from build123d import *

# Parameters (mm, degrees)
SKETCH3_W           = 302.8427
SKETCH3_H           = 302.8427
BOSS_EXTRUDE1_DEPTH = 790
BOSS_EXTRUDE1_DRAFT = -3
SKETCH6_W           = 200
SKETCH6_H           = 200
CUT_EXTRUDE3_DEPTH  = 790
CUT_EXTRUDE3_DRAFT  = 3
SKETCH7_W           = 250
SKETCH7_H           = 250
SKETCH7_R           = 2.5
SKETCH7_W_2         = 200
SKETCH7_H_2         = 200
BOSS_EXTRUDE2_DEPTH = 5
SKETCH8_W           = 332.804291268
SKETCH8_H           = 332.804291268
SKETCH8_R           = 2.5
SKETCH8_W_2         = 282.804291268
SKETCH8_H_2         = 282.804291268
BOSS_EXTRUDE3_DEPTH = 5


with BuildPart() as part:
    # Sketch3 → Boss-Extrude1 (with draft: the straight prism first)
    with BuildSketch(Plane.XY.offset(790)):
        Rectangle(SKETCH3_W, SKETCH3_H)
    extrude(amount=-BOSS_EXTRUDE1_DEPTH)
    # Boss-Extrude1: the draft: its side faces are tilted about the plane it starts from
    boss_extrude1_sides = [part.faces().sort_by_distance(p)[0] for p in [
        (0, 151.42135, 395),
        (-151.42135, 0, 395),
        (0, -151.42135, 395),
        (151.42135, 0, 395),
    ]]
    draft(boss_extrude1_sides, Plane.XY.offset(790), BOSS_EXTRUDE1_DRAFT)


with BuildPart() as cut_extrude3_tool:
    # Sketch6 → Cut-Extrude3 (with draft: the straight prism first)
    with BuildSketch(Plane(origin=(0, 0, 0), x_dir=(-1, 0, 0), z_dir=(0, 0, -1))):
        Rectangle(SKETCH6_W, SKETCH6_H)
    extrude(amount=-CUT_EXTRUDE3_DEPTH)
    # Cut-Extrude3: the draft: its side faces are tilted about the plane it starts from
    cut_extrude3_sides = [cut_extrude3_tool.faces().sort_by_distance(p)[0] for p in [
        (0, -100, 395),
        (-100, 0, 395),
        (0, 100, 395),
        (100, 0, 395),
    ]]
    draft(cut_extrude3_sides, Plane(origin=(0, 0, 0), x_dir=(-1, 0, 0), z_dir=(0, 0, -1)), CUT_EXTRUDE3_DRAFT)


with BuildPart() as part_1:
    add(part.part)

    # Cut-Extrude3: cut by cut_extrude3_tool
    add(cut_extrude3_tool.part, mode=Mode.SUBTRACT)

    # Sketch7 → Boss-Extrude2 (add)
    with BuildSketch(Plane(origin=(0, 0, 0), x_dir=(-1, 0, 0), z_dir=(0, 0, -1))):
        Rectangle(SKETCH7_W, SKETCH7_H)
        with Locations((0, -117.5)):
            Circle(SKETCH7_R, mode=Mode.SUBTRACT)
        with Locations((-117.509602183, 117.509602183)):
            Circle(SKETCH7_R, mode=Mode.SUBTRACT)
        with Locations(Location((117.509602183, -117.509602183, 0), (0, 0, 180))):
            Circle(SKETCH7_R, mode=Mode.SUBTRACT)
        with Locations(Location((-117.5, 0, 0), (0, 0, 180))):
            Circle(SKETCH7_R, mode=Mode.SUBTRACT)
        with Locations((-117.509602183, -117.509602183)):
            Circle(SKETCH7_R, mode=Mode.SUBTRACT)
        with Locations(Location((117.509602183, 117.509602183, 0), (0, 0, 180))):
            Circle(SKETCH7_R, mode=Mode.SUBTRACT)
        with Locations((117.5, 0)):
            Circle(SKETCH7_R, mode=Mode.SUBTRACT)
        with Locations((-1.21803637, 117.509602183)):
            Circle(SKETCH7_R, mode=Mode.SUBTRACT)
        Rectangle(SKETCH7_W_2, SKETCH7_H_2, mode=Mode.SUBTRACT)
    extrude(amount=-BOSS_EXTRUDE2_DEPTH)

    # Sketch8 → Boss-Extrude3 (add)
    with BuildSketch(Plane.XY.offset(790)):
        Rectangle(SKETCH8_W, SKETCH8_H)
        with Locations((-158.911747817, 0)):
            Circle(SKETCH8_R, mode=Mode.SUBTRACT)
        with Locations((-158.911747817, 158.911747817)):
            Circle(SKETCH8_R, mode=Mode.SUBTRACT)
        with Locations(Location((158.911747817, -158.911747817, 0), (0, 0, 180))):
            Circle(SKETCH8_R, mode=Mode.SUBTRACT)
        with Locations(Location((0, -158.911747817, 0), (0, 0, 180))):
            Circle(SKETCH8_R, mode=Mode.SUBTRACT)
        with Locations((158.911747817, 158.911747817)):
            Circle(SKETCH8_R, mode=Mode.SUBTRACT)
        with Locations((0, 158.911747817)):
            Circle(SKETCH8_R, mode=Mode.SUBTRACT)
        with Locations(Location((-158.911747817, -158.911747817, 0), (0, 0, 180))):
            Circle(SKETCH8_R, mode=Mode.SUBTRACT)
        with Locations((158.911747817, 0)):
            Circle(SKETCH8_R, mode=Mode.SUBTRACT)
        Rectangle(SKETCH8_W_2, SKETCH8_H_2, mode=Mode.SUBTRACT)
    extrude(amount=-BOSS_EXTRUDE3_DEPTH)


solid = part_1.part
The listing builds one solid part. Answer for the finished solid, in the listing's coordinates (mm). A direction names the side the tool comes from. Give positions to 0.01 mm unless a question says otherwise; leave off trailing zeros. Write each loop counter-clockwise with the first axis right and the second up, starting at its lowest first coordinate (ties: lowest second). Pieces come first, ordered by that corner, then holes. Notation, with made-up numbers: (1.5, 75.5) -> (18.5, 75.5) arc R29 cw to (18.5, 99.5) -> close; hole circle Ø8 at (14.25, 41.25). An arc over 180 degrees is marked (long way). One line per question, with ' | ' between items. Start each with the question number.
1. Section A-A (y = 35) is taken. Determine the outline of the cut face in (x, z), plus the area to 3 significant figures.
2. Section C-C (z = 644) is taken. Determine the outline of the cut face in (x, y).
3. For a pull along Z with two mould halves and no side action, classify faces 1 (the flat face through (-120.544, -1.98, 392.005)), 2 (the flat face through (113, 2, 0)), 3 (the flat face through (-2.116, -131.006, 400.46)) as pulls with the +Z half, pulls with the -Z half, needs draft (parallel to the pull), parting line crosses it, or undercut.
4. Find the intervals of material crossed by probe 1 along Y at (x, z) = (0, 787.8); probe 2 along X at (y, z) = (-32.5, 209); probe 3 along X at (y, z) = (-4.5, 536), in increasing order.
5. For faces 4 (the flat face through (1.98, 120.544, 392.005)), 5 (the flat face through (-2.116, 131.006, 400.46)), 6 (the flat face through (1, 112, 5)), 7 (the flat face through (131.006, -2.116, 400.46)), 8 (the flat face through (-161, 13, 785)), determine the directions among +Z, -Z, +X, -X, +Y, -Y from which every point of the face is accessible in a straight line to the end or side of a thin tool.
6. Given pin 1 Ø4 at (x, z) = (131.5, 556.5) entering from +Y; pin 2 Ø3 at (x, y) = (-158.91, -158.91) entering from +Z; pin 3 Ø6 at (x, y) = (-158.91, 158.91) entering from -Z; pin 4 Ø4 at (x, z) = (42, 2.5) entering from -Y, each flat-ended and moving along its own axis, determine where each tip first touches the part or whether it passes through.
7. Section D-D (z = 207.5) is taken. Determine the outline of the cut face in (x, y), plus the area to 3 significant figures.
Response values:
1) outline: (-166.4, 785) -> (-151.16, 785) -> (-110.28, 5) -> (-125, 5) -> (-125, 0) -> (-100, 0) -> (-100, 5) -> (-100.26, 5) -> (-141.4, 790) -> (-166.4, 790) -> close; (100, 0) -> (125, 0) -> (125, 5) -> (110.28, 5) -> (151.16, 785) -> (166.4, 785) -> (166.4, 790) -> (141.4, 790) -> (100.26, 5) -> (100, 5) -> close | area: 16,100 mm2
2) outline: (-143.77, -143.77) -> (143.77, -143.77) -> (143.77, 143.77) -> (-143.77, 143.77) -> close; hole (-133.75, -133.75) -> (133.75, -133.75) -> (133.75, 133.75) -> (-133.75, 133.75) -> close
3) face 1: pulls with the +Z half | face 2: pulls with the -Z half | face 3: undercut
4) probe 1: -166.4 to -161.41, -156.41 to -141.29, 141.29 to 156.41, 161.41 to 166.4 | probe 2: -120.97 to -110.95, 110.95 to 120.97 | probe 3: -138.11 to -128.09, 128.09 to 138.11
5) face 4: +Z | face 5: +X, -X, +Y | face 6: none | face 7: +X, +Y, -Y | face 8: -Z
6) pin 1: y = 139.29 | pin 2: through | pin 3: z = 785 | pin 4: y = -125
7) outline: (-120.89, -120.89) -> (120.89, -120.89) -> (120.89, 120.89) -> (-120.89, 120.89) -> close; hole (-110.87, -110.87) -> (110.87, -110.87) -> (110.87, 110.87) -> (-110.87, 110.87) -> close | area: 9,290 mm2
